Build history of the part. All positions in model axes, mm. Face numbers are marked on the shaded views. A direction names the side the tool comes from. Give positions to 0.01 mm unless a question says otherwise; leave off trailing zeros. Write each loop counter-clockwise with the first axis right and the second up, starting at its lowest first coordinate (ties: lowest second). Pieces come first, ordered by that corner, then holes.
from build123d import *

# Parameters (mm, degrees)
ESQUISSE1_W             = 17
ESQUISSE1_H             = 5
BOSS_EXTRU_1_DEPTH      = 24
BOSS_EXTRU_2_DEPTH      = 24
CONG_1_R                = 4
CONG_2_R                = 8
CONG_3_R                = 3
ESQUISSE3_W             = 24
ESQUISSE3_H             = 5
BOSS_EXTRU_3_DEPTH      = 20
ESQUISSE4_R             = 2.1
ENL_V_MAT_EXTRU_1_DEPTH = 10
CONG_4_R                = 3
ESQUISSE5_R             = 2.25
ENL_V_MAT_EXTRU_2_DEPTH = 4


with BuildPart() as part:
    # Esquisse1 → Boss.-Extru.1 (new body)
    with BuildSketch(Plane.XY):
        with Locations((1.940369129, 2.5)):
            Rectangle(ESQUISSE1_W, ESQUISSE1_H)
    extrude(amount=BOSS_EXTRU_1_DEPTH)

    # Esquisse2 → Boss.-Extru.2 (add)
    with BuildSketch(Plane.XY.offset(24)):
        Polygon((-18.723069156, 0.535871193), (-3.080508445, -7.355303518), (-0.501566554, -3.056100904), (-16.471058056, 5), align=None)
        Polygon((-6.559630871, 0), (-6.559630871, 5), (-16.471058056, 5), align=None)
    extrude(amount=-BOSS_EXTRU_2_DEPTH)

    # Congé1
    cong_1_edges = [part.edges().sort_by_distance(p)[0] for p in [
        (-0.501566554, -3.056100904, 12),
    ]]
    fillet(cong_1_edges, radius=CONG_1_R)

    # Congé2
    cong_2_edges = [part.edges().sort_by_distance(p)[0] for p in [
        (-16.471058056, 5, 12),
    ]]
    fillet(cong_2_edges, radius=CONG_2_R)

    # Congé3
    cong_3_edges = [part.edges().sort_by_distance(p)[0] for p in [
        (-6.559630871, 0, 12),
    ]]
    fillet(cong_3_edges, radius=CONG_3_R)

    # Esquisse3 → Boss.-Extru.3 (add)
    with BuildSketch(Plane(origin=(10.440369129, 0, 0), x_dir=(0, 0, -1), z_dir=(1, 0, 0))):
        with Locations((-12, 2.5)):
            Rectangle(ESQUISSE3_W, ESQUISSE3_H)
    extrude(amount=BOSS_EXTRU_3_DEPTH)

    # Esquisse4 → Enlèv. mat.-Extru.1 (cut)
    with BuildSketch(Plane(origin=(0, 5, 0), x_dir=(1, 0, 0), z_dir=(0, 1, 0))):
        with Locations((8.440369129, -8)):
            Circle(ESQUISSE4_R)
        with Locations((24.440369129, -8)):
            Circle(ESQUISSE4_R)
        with Locations((8.440369129, -16)):
            Circle(ESQUISSE4_R)
        with Locations((24.440369129, -16)):
            Circle(ESQUISSE4_R)
    extrude(amount=-ENL_V_MAT_EXTRU_1_DEPTH, mode=Mode.SUBTRACT)

    # Congé4
    cong_4_edges = [part.edges().sort_by_distance(p)[0] for p in [
        (30.440369129, 2.5, 0),
        (30.440369129, 2.5, 24),
    ]]
    fillet(cong_4_edges, radius=CONG_4_R)

    # Esquisse5 → Enlèv. mat.-Extru.2 (cut)
    with BuildSketch(Plane(origin=(-3.582711985, -7.101957793, 0), x_dir=(0.892825761, -0.45040222, 0), z_dir=(-0.45040222, -0.892825761, 0))):
        with Locations((-12.147654158, 8.05)):
            Circle(ESQUISSE5_R)
        with Locations((-12.147654158, 15.95)):
            Circle(ESQUISSE5_R)
        with Locations((-4.247654158, 15.95)):
            Circle(ESQUISSE5_R)
        with Locations((-4.247654158, 8.05)):
            Circle(ESQUISSE5_R)
    extrude(amount=-ENL_V_MAT_EXTRU_2_DEPTH, mode=Mode.SUBTRACT)


solid = part.part
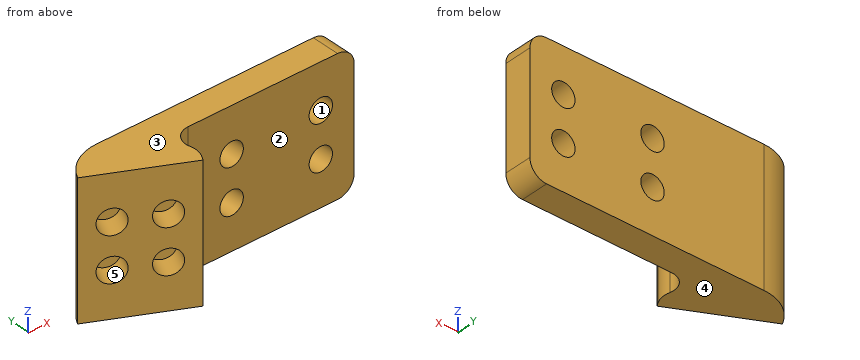
(1) Saw through at B-B, the plane z = 15. Give the number of separate pieces and of enclosed holes in the cut face, plus the area to 3 significant figures.
(2) Saw through at A-A, the plane x = 23. List the corners of the cut face in (y, z), plus the area to 3 significant figures.
(3) Probe line 1 (Z direction, x = 23, y = 4); line 2 (X direction, y = 1.25, z = 14.75); line 3 (X direction, y = 2.1, z = 8). List the from-to ranges inside material, lowest first.
(4) Mould opens along Z. For the marked faces 3, 4 and 5 say: +Z half, -Z half, draft (parallel to the pull), parting line (faces both ways), or undercut.
(5) 3-axis set-ups, long thin cutter, end or side, ignore diameter. For the marked faces 1 and 2: which of +Z, -Z, +X, -X, +Y, -Y reach the whole face in a straight line?
(6) Drop flat-ended pins along their axis: pin 1 (12 mm diameter, centred on x = 18.5, z = 15.5, fed in from -Y); pin 2 (2 mm diameter, centred on y = 0, z = 18, fed in from -X); pin 3 (3.5 mm diameter, centred on x = 8.44, z = 16, fed in from -Y); pin 4 (1.5 mm diameter, centred on y = 1.5, z = 19.5, fed in from -X). Give the stop position or say it passes through.
Computed values:
1. separate pieces: 3
1. enclosed holes: 0
1. area: 228 mm2
2. outline: (0, 0) - (5, 0) - (5, 6.47) - (0, 6.47) - close; (0, 9.53) - (5, 9.53) - (5, 14.47) - (0, 14.47) - close; (0, 17.53) - (5, 17.53) - (5, 24) - (0, 24) - close
2. area: 89.4 mm2
3. line 1: z = 0 to 6.47, 9.53 to 14.47, 17.53 to 24
3. line 2: x = -18.32 to -15.11, -11.26 to 6.75, 10.13 to 22.75, 26.13 to 30.44
3. line 3: x = -17.71 to -15.07, -12.94 to 6.34, 10.54 to 22.34, 26.54 to 30.44
4. face 3: +Z half
4. face 4: -Z half
4. face 5: undercut
5. face 1: +Y, -Y
5. face 2: +Z, -Z, +X, -Y
6. pin 1: stops at y = 0
6. pin 2: stops at x = -18.72
6. pin 3: passes through
6. pin 4: stops at x = -18.61
